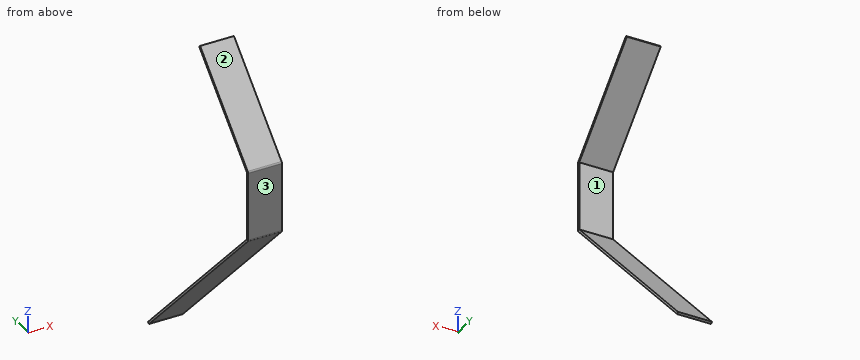
Autodesk Inventor part; units mm, degrees
ref_plane "YZ Plane" through (0, 0, 0) normal (1, 0, 0) x (0, 1, 0)
ref_plane "XZ Plane" through (0, 0, 0) normal (0, 1, 0) x (-1, 0, 0)
ref_plane "XY Plane" through (0, 0, 0) normal (0, 0, 1) x (1, 0, 0)
sketch "Sketch1" plane through (0, 0, 0) normal (0, 1, 0) x (-1, 0, 0)
  line L0 (12.7, 161.925) -> (-12.7, 161.925)
  line L1 (-12.7, 161.925) -> (-12.7, -161.925)
  line L2 (-12.7, -161.925) -> (12.7, -161.925)
  line L3 (12.7, -161.925) -> (12.7, 161.925)
  line L4 (12.7, 161.925) -> (-12.7, -161.925) construction
  line L5 (-12.7, 161.925) -> (12.7, -161.925) construction
  point P0 (0, 0)
  dimension "d0" = 25.4
  dimension "d1" = 323.85
extrude "Extrusion1" add sketch "Sketch1" along normal blind 1.5875
sketch "Sketch2" plane through (0, 1.5875, 0) normal (0, 1, 0) x (1, 0, 0)
  line L0 (-12.7, -161.925) -> (12.7, -161.925)
  line L1 (-43.2277, -22.225) -> (46.1542, -22.225)
  point P0 (0, 0)
  dimension "d4" = 139.7
bend part "Bend Part1" radius 0.3234 angle 45 line through (-43.2277, 1.5875, 22.225) along (1, 0, 0) centre toward (0, 1, 0) moving side (0, 0, -1) both sides yes
sketch "Sketch4" plane through (-12.7, 1.6121, 22.3488) normal (0, 0.9238795, -0.3826834) x (1, 0, 0)
  line L0 (25.4, 0) -> (0, 0)
  line L1 (25.4, -139.573) -> (25.4, 0)
  line L2 (-18.5864, -50.8) -> (43.4016, -50.8)
  point P0 (12.7, 21.2645)
  dimension "d8" = 50.8
bend part "Bend Part2" radius 0.3234 angle 45 line through (-31.2864, 21.0524, 69.2818) along (1, 0, 0) centre toward (0, 0.9238795, -0.3826834) moving side (0, -0.3826834, -0.9238795) both sides yes
properties part number "finger" material "Polycarbonate, Clear"
Verification items for the finished model (mm, model axes). Face numbers are marked on the shaded views. Round coordinates to 2 decimals unless told otherwise and drop trailing zeros. Write each loop counter-clockwise with the first axis right and the second up, starting at its lowest first coordinate (ties: lowest second). Pieces come first, ordered by that corner, then holes. Notation, with made-up numbers: (30.25, 9.25) -> (82.25, 9.25) arc R26 ccw to (82.25, 40.25) -> close; hole circle Ø2 at (-6.75, 46). An arc over 180 degrees is marked (long way). Write each question's results on one line, items separated by ' | '.
Q1. Sectioned sample at D-D, the plane z = 76. Record the boundary of the cut face in (x, y).
Derived:
outline: (-12.7, 25.49) -> (12.7, 25.49) -> (12.7, 27.74) -> (-12.7, 27.74) -> close
Q2. Draft check along Z on the marked faces 1, 2 and 3. Enter one of: released by +Z, released by -Z, zero draft, split by the parting line, or undercut.
Derived:
face 1: undercut | face 2: released by +Z | face 3: zero draft
Q3. Go/stop test with flat-tipped pins: pin 1 Ø6 at (x, y) = (-7, 56.5) entering from -Z; pin 2 Ø12 at (x, y) = (6.5, 61.5) entering from +Z; pin 3 Ø8 at (x, y) = (9.5, 119) entering from +Z. Record where each tip stops, or that it passes through.
Derived:
pin 1: stops at z = -22.37 | pin 2: stops at z = 118.01 | pin 3: stops at z = -75.62
Q4. Thickness scan on probe 1 along Y at (x, z) = (3, 67.5); probe 2 along Z at (x, y) = (-3, 60); probe 3 along Y at (x, z) = (-8, -41). Record the ranges inside material, lowest first.
Derived:
probe 1: y = 19.44 to 21.03 | probe 2: z = -22.87 to -20.62, 108.26 to 110.51 | probe 3: y = 78.13 to 80.38
Q5. Sectioned sample at C-C, the plane y = 131. Record the boundary of the cut face in (x, z), and give its area (3 significant figures).
Derived:
outline: (-12.7, -93.87) -> (12.7, -93.87) -> (12.7, -91.62) -> (-12.7, -91.62) -> close | area: 57.0 mm²
Q6. Sectioned sample at A-A, the plane x = 4.75. Record the boundary of the cut face in (y, z).
Derived:
outline: (19.44, 18.49) arc R1.91 ccw to (20, 17.13) -> (150.12, -112.99) -> (151.25, -111.87) -> (21.12, 18.26) arc R0.32 cw to (21.03, 18.49) -> (21.03, 69.16) arc R0.32 cw to (21.12, 69.39) -> (83.8, 132.07) -> (82.68, 133.19) -> (20, 70.51) arc R1.91 ccw to (19.44, 69.16) -> close
Q7. Sectioned sample at B-B, the plane y = 51. Record the boundary of the cut face in (x, z).
Derived:
outline: (-12.7, -13.87) -> (12.7, -13.87) -> (12.7, -11.62) -> (-12.7, -11.62) -> close; (-12.7, 99.26) -> (12.7, 99.26) -> (12.7, 101.51) -> (-12.7, 101.51) -> close
